Autodesk Inventor part; units mm, degrees
ref_plane "YZ Plane" through (0, 0, 0) normal (1, 0, 0) x (0, 1, 0)
ref_plane "XZ Plane" through (0, 0, 0) normal (0, 1, 0) x (-1, 0, 0)
ref_plane "XY Plane" through (0, 0, 0) normal (0, 0, 1) x (1, 0, 0)
sketch "Sketch1" plane through (0, 0, 0) normal (0, 0, 1) x (1, 0, 0)
  line L0 (-70, -135) -> (70, -135)
  line L1 (70, -135) -> (70, 135)
  line L2 (70, 135) -> (-70, 135)
  line L3 (-70, 135) -> (-70, -135)
  line L4 (-70, -135) -> (70, 135) construction
  line L5 (70, -135) -> (-70, 135) construction
  point P0 (0, 0)
  dimension "d0" = 140
  dimension "d1" = 270
extrude "Plate1" add sketch "Sketch1" along normal blind 2
sketch "Sketch3" plane through (70, 133, 2) normal (0, 1, 0) x (-1, 0, 0)
  line L0 (140, 0) -> (0, 0)
  line L1 (0, 0) -> (0, -50)
  line L2 (0, -50) -> (140, -50)
  line L3 (140, -50) -> (140, 0)
edge flange "Flange1" height 50 angle 90 thickness 2 bend radius 2.75 thickness toward (0, 1, 0) relief round relief width 2 relief depth 1 corner gap 2.75 corner form 0 edges at (0, 135, 0) (0, -135, 0) wall of the first edge with corners at (-70, 133, 2) (70, 133, 2) (70, 133, -48) (-70, 133, -48)
bend "Bend1"
corner "Corner1"
sketch "Sketch4" plane through (-70, 133, -46) normal (0, 0, -1) x (-1, 0, 0)
  line L0 (-140, 0) -> (0, 0)
  line L1 (0, 0) -> (0, 15)
  line L2 (0, 15) -> (-140, 15)
  line L3 (-140, 15) -> (-140, 0)
edge flange "Flange2" height 15 angle 90 thickness 2 bend radius 2.75 thickness toward (0, 0, -1) relief round relief width 2 relief depth 1 corner gap 2.75 corner form 0 edges at (0, 135, -48) (0, -135, -48) wall of the first edge with corners at (70, 133, -46) (-70, 133, -46) (-70, 148, -46) (70, 148, -46)
bend "Bend2"
corner "Corner2"
equation "\"d2\" = Thickness"
equation "\"d6\" = BendReliefWidth"
equation "\"d7\" = BendReliefDepth"
equation "\"d8\" = MinimumRemnant"
equation "\"d9\" = TransitionRadius"
equation "\"d12\" = BendRadius"
equation "\"d13\" = CornerReliefSize"
equation "\"d14\" = GapSize"
equation "\"d15\" = JacobiRadiusSize"
equation "\"d16\" = BendReliefWidth"
equation "\"d17\" = BendReliefDepth"
equation "\"d18\" = MinimumRemnant"
equation "\"d19\" = TransitionRadius"
equation "\"d22\" = BendRadius"
equation "\"d23\" = CornerReliefSize"
equation "\"d24\" = GapSize"
equation "\"d25\" = JacobiRadiusSize"
equation "\"BendReliefWidth\" = Thickness"
equation "\"BendReliefDepth\" = 0.5 * Thickness"
equation "\"CornerReliefSize\" = 4 * Thickness"
equation "\"MinimumRemnant\" = 2 * Thickness"
equation "\"TransitionRadius\" = BendRadius"
equation "\"JacobiRadiusSize\" = BendRadius"
equation "\"GapSize\" = Thickness"
properties part number "BSH pollar 5" material "Stainless Steel"
Can you work these out from the model? Positions are in its coordinate system, mm. A direction names the side the tool comes from. Coordinates: 2 decimals unless noted, no trailing zeros. Write each loop counter-clockwise with the first axis right and the second up, starting at its lowest first coordinate (ties: lowest second). Pieces come first, ordered by that corner, then holes. Notation, with made-up numbers: (67, -17) - (74, -17) arc R11 cw to (74, -8) - close; hole circle Ø5 at (2.25, 16.25). An arc over 180 degrees is marked (long way). Return JSON: item names as keys, results as strings. Group by question number.
Item 1: If we section it at C-C (y = -104): Write out the boundary of the cut face in (x, z), then the cut area to 3 significant figures.
Item 2: I'm going to push flat-ended pins straight in: pin 1 Ø11.5 at (x, y) = (-6, 142.5) entering from +Z; pin 2 Ø3 at (x, z) = (31.5, -16.5) entering from -Y; pin 3 Ø8 at (x, y) = (-30.5, -145) entering from +Z. Where does each tip first touch, or does it pass through?
Item 3: If we section it at B-B (x = 30): Write out the boundary of the cut face in (y, z), then the cut area to 3 significant figures.
Item 4: If we section it at A-A (z = -26.5): Write out the boundary of the cut face in (x, y).
Item 5: Which directions (+Z, -Z, +X, -X, +Y, -Y) give clear straight access to the entire face, cutting with the end or side of a thin tool? Please do faces 5 (the face through (1, -143, -46)), 6 (the face through (70, 1, 1)), 7 (the face through (1, 133, -23)), 8 (the face through (-1, 143, -46)).
Item 6: We'd pull the mould along Y, two halves only. Please class faces 1 (the face through (-1, -135, -23)), 2 (the face through (-1, -133, -23)), 3 (the face through (-1, 2, 0)), 4 (the face through (-1, 2, 2)): pulls with the +Y half, pulls with the -Y half, needs draft (parallel to the pull), parting line crosses it, or undercut.
Item 7: Please list where these lines run through material, in increasing order: probe 1 along Y at (x, z) = (1, -15.5); probe 2 along Z at (x, y) = (24.5, -112.5); probe 3 along Y at (x, z) = (-36, -45).
Return value:
{
 "1": {"outline": "(-70, 0) - (70, 0) - (70, 2) - (-70, 2) - close", "area": "280 mm^2"},
 "2": {"pin 1": "stops at z = -45.81", "pin 2": "stops at y = -135", "pin 3": "stops at z = -46"},
 "3": {"outline": "(-148, -48) - (-137.75, -48) arc R4.75 ccw to (-133, -43.25) - (-133, -2.75) arc R2.75 cw to (-130.25, 0) - (130.25, 0) arc R2.75 cw to (133, -2.75) - (133, -43.25) arc R4.75 ccw to (137.75, -48) - (148, -48) - (148, -46) - (137.75, -46) arc R2.75 cw to (135, -43.25) - (135, -2.75) arc R4.75 ccw to (130.25, 2) - (-130.25, 2) arc R4.75 ccw to (-135, -2.75) - (-135, -43.25) arc R2.75 cw to (-137.75, -46) - (-148, -46) - close", "area": "771 mm^2"},
 "4": {"outline": "(-70, -135) - (70, -135) - (70, -133) - (-70, -133) - close; (-70, 133) - (70, 133) - (70, 135) - (-70, 135) - close"},
 "5": {"face 5": "+Z, +X, -X, -Y", "face 6": "+Z, -Z, +X, +Y, -Y", "face 7": "-Z, +X, -X", "face 8": "+Z, +X, -X, +Y"},
 "6": {"face 1": "pulls with the -Y half", "face 2": "undercut", "face 3": "undercut", "face 4": "needs draft"},
 "7": {"probe 1": "y = -135 to -133, 133 to 135", "probe 2": "z = 0 to 2", "probe 3": "y = -135.63 to -133.33, 133.33 to 135.63"}
}
